Could you check a few things on this model? Use its own coordinates, in mm. Round coordinates to 2 decimals unless told otherwise and drop trailing zeros. Order: outer loops, then holes, each group sorted by start corner. A loop starts at its lowest first (then second) coordinate and runs counter-clockwise, first axis right, second up. Notation, with made-up numbers: (11.25, 28.5) - (37.25, 28.5) arc R15 ccw to (37.25, 34.5) - close; hole circle Ø8 at (-22.5, 0.5). An arc over 180 degrees is marked (long way). Use one line per item in the form item = value.
from build123d import *

# Parameters (mm, degrees)
F0_R     = 7.14375
F1_DEPTH = 3.175


with BuildPart() as f1:
    # F0 (on Front) → F1 (new body)
    with BuildSketch(Plane.XZ):
        with BuildLine():
            add(Edge.make_bspline(
                [(82.926092, 165.021802), (92.632547, 184.53142), (64.966619, 200.063169), (50.946968, 185.499491)],
                knots=[0, 0, 0, 0, 37.973677, 37.973677, 37.973677, 37.973677], degree=3))
            Line((50.946968, 185.499491), (-105.013265, 36.552987))
            add(Edge.make_bspline(
                [(-105.013265, 36.552987), (-121.657088, 21.448022), (-114.376582, 2.033332), (-94.6206, 1.375155)],
                knots=[0, 0, 0, 0, 36.680886, 36.680886, 36.680886, 36.680886], degree=3))
            Line((-94.6206, 1.375155), (-31.048113, 1.375155))
            add(Edge.make_bspline(
                [(-31.048113, 1.375155), (-22.642167, 2.033332), (-20.215331, 3.24675), (-15.296232, 9.48368)],
                knots=[0, 0, 0, 0, 17.716376, 17.716376, 17.716376, 17.716376], degree=3))
            Line((-15.296232, 9.48368), (82.926092, 165.021802))
        make_face()
        with Locations((-94.318171, 20.425155)):
            Circle(F0_R, mode=Mode.SUBTRACT)
        with Locations((-30.818171, 20.582018)):
            Circle(F0_R, mode=Mode.SUBTRACT)
        with Locations((65.422429, 172.982018)):
            Circle(F0_R, mode=Mode.SUBTRACT)
    extrude(amount=F1_DEPTH)


solid = f1.part
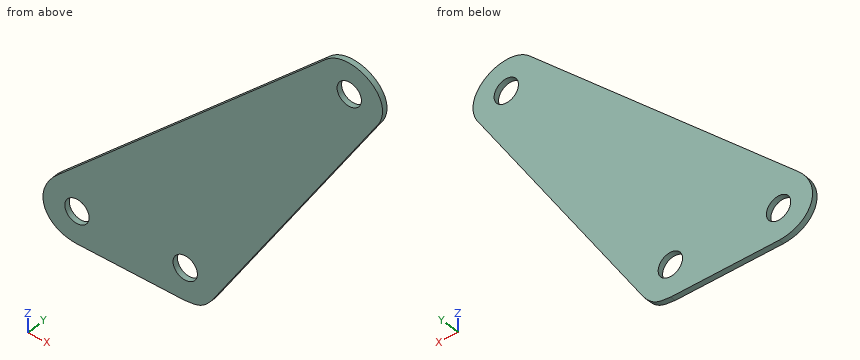
Item 1: Imagine slicing it at C-C on z = 154.5. Please give me the cut outline in (x, y) (3 decimals), plus the area to 3 significant figures.
Found:
outline = (18.488, -3.175) - (76.282, -3.175) - (76.282, 0) - (18.488, 0) - close
area = 183 mm2
Item 2: I need wall thicknesses on L1, parallel to X at y = -1.3, z = 20; L2, parallel to Z at x = 23, y = -1.8; L3, parallel to X at y = -0.2, z = 89. Which ranges of each line are inside material? Lowest first, please.
Found:
L1 = -114.2 to -101.45, -87.19 to -37.94, -23.7 to -8.66
L2 = 70.13 to 158.81
L3 = -50.1 to 34.92
Item 3: Will these pins go through, and if not, where does the flat tip stop? P1, Ø13, axis at x = 65.42, z = 172.98, coming from the -Y side; P2, Ø1, axis at y = -2.5, z = 141, coming from the +X side; P3, Ø1, axis at x = -83, y = -1.5, coming from the +Z side.
Found:
P1 = through
P2 = 68.07
P3 = 58.05
Item 4: Imagine slicing it at A-A on x = -90. Please give me the cut outline in (y, z) (3 decimals).
Found:
outline = (-3.175, 1.375) - (0, 1.375) - (0, 14.734) - (-3.175, 14.734) - close; (-3.175, 26.116) - (0, 26.116) - (0, 50.891) - (-3.175, 50.891) - close
Item 5: Imagine slicing it at B-B on z = 24. State how many separate pieces and enclosed holes the cut face has, plus the area to 3 significant figures.
Found:
separate_pieces = 3
enclosed_holes = 0
area = 262 mm2
